```python
from build123d import *

# Parameters (mm, degrees)
SKETCH1_R           = 1.875
BOSS_EXTRUDE1_DEPTH = 15
SKETCH2_W           = 35
SKETCH2_H           = 2.286
CUT_EXTRUDE1_DEPTH  = 1.778
SKETCH7_W           = 23.625
SKETCH7_H           = 2.286
CUT_EXTRUDE6_DEPTH  = 5
SKETCH3_R           = 3.302
CUT_EXTRUDE2_DEPTH  = 3.556
SKETCH4_R           = 3.302
CUT_EXTRUDE3_DEPTH  = 3.302
SKETCH5_W           = 35
SKETCH5_H           = 15
CUT_EXTRUDE4_DEPTH  = 0.762
CUT_EXTRUDE5_DEPTH  = 73.293856534
FILLET1_R           = 3
FILLET2_R           = 1


with BuildPart() as part:
    # Sketch1 → Boss-Extrude1 (new body)
    with BuildSketch(Plane(origin=(0, 0, 0), x_dir=(1, 0, 0), z_dir=(0, 1, 0))):
        with BuildLine():
            Line((-60.8, 0), (0, 0))
            Line((0, 0), (0, 35))
            Line((0, 35), (-16.036868781, 35))
            Line((-16.036868781, 35), (-16.036868781, 15))
            Line((-16.036868781, 15), (-60.8, 15))
            ThreePointArc((-60.8, 15), (-61.45243439, 7.5), (-60.8, 0))
        make_face()
        with Locations(Location((-8.01843439, 7.5, 0), (0, 0, 270))):
            Circle(SKETCH1_R, mode=Mode.SUBTRACT)
    extrude(amount=BOSS_EXTRUDE1_DEPTH)

    # Sketch2 → Cut-Extrude1 (cut)
    with BuildSketch(Plane(origin=(0, 0, 0), x_dir=(0, 0, -1), z_dir=(1, 0, 0))):
        with BuildLine():
            Line((22.486, 12.716), (22.486, 15))
            Line((22.486, 15), (0, 15))
            Line((0, 15), (0, 4.043897552))
            Line((0, 4.043897552), (18.893897552, 4.043897552))
            ThreePointArc((18.893897552, 4.043897552), (27.179308025, 5.691968164), (22.486, 12.716))
        make_face()
        with Locations((17.5, 1.143)):
            Rectangle(SKETCH2_W, SKETCH2_H)
    extrude(amount=-CUT_EXTRUDE1_DEPTH, mode=Mode.SUBTRACT)

    # Sketch7 → Cut-Extrude6 (cut)
    with BuildSketch(Plane(origin=(-1.778, 0, 0), x_dir=(0, 0, -1), z_dir=(1, 0, 0))):
        with Locations((23.1875, 1.143)):
            Rectangle(SKETCH7_W, SKETCH7_H)
    extrude(amount=-CUT_EXTRUDE6_DEPTH, mode=Mode.SUBTRACT)

    # Sketch3 → Cut-Extrude2 (cut)
    with BuildSketch(Plane(origin=(-1.778, 0, 0), x_dir=(0, 0, -1), z_dir=(1, 0, 0))):
        with Locations((22.486, 7.636)):
            Circle(SKETCH3_R)
    extrude(amount=-CUT_EXTRUDE2_DEPTH, mode=Mode.SUBTRACT)

    # Sketch4 → Cut-Extrude3 (cut)
    with BuildSketch(Plane(origin=(0, 0, -15), x_dir=(-1, 0, 0), z_dir=(0, 0, -1))):
        with Locations((43.57843439, 7.5)):
            Circle(SKETCH4_R)
    extrude(amount=-CUT_EXTRUDE3_DEPTH, mode=Mode.SUBTRACT)

    # Sketch5 → Cut-Extrude4 (cut)
    with BuildSketch(Plane(origin=(0, 0, 0), x_dir=(0, 0, -1), z_dir=(1, 0, 0))):
        with Locations((17.5, 7.5)):
            Rectangle(SKETCH5_W, SKETCH5_H)
    extrude(amount=-CUT_EXTRUDE4_DEPTH, mode=Mode.SUBTRACT)

    # Sketch6 → Cut-Extrude5 (cut, through all)
    with BuildSketch(Plane(origin=(0, 15, 0), x_dir=(1, 0, 0), z_dir=(0, 1, 0))):
        with BuildLine():
            Line((-8.262, 0), (-0.762, 0))
            Line((-0.762, 0), (-0.762, 7.5))
            ThreePointArc((-0.762, 7.5), (-2.958699141, 2.196699141), (-8.262, 0))
        make_face()
    extrude(amount=-CUT_EXTRUDE5_DEPTH, mode=Mode.SUBTRACT)

    # Fillet1
    fillet1_edges = [part.edges().sort_by_distance(p)[0] for p in [
        (-60.8, 7.5, 0),
        (-60.8, 7.5, -15),
        (-16.036868781, 7.5, -15),
        (-16.036868781, 7.5, -35),
        (-0.762, 8.643, -35),
    ]]
    fillet(fillet1_edges, radius=FILLET1_R)

    # Fillet2
    fillet2_edges = [part.edges().sort_by_distance(p)[0] for p in [
        (-1.778, 0, -7.552841941),
        (-4.521670528, 15, -0.99923578),
        (-4.521670528, 0, -0.99923578),
        (-61.45243439, 0, -7.5),
        (-61.45243439, 15, -7.5),
        (-33.231623045, 0, 0),
        (-38.619057435, 0, -15),
        (-16.036868781, 0, -25),
        (-15.158189125, 0, -34.121320344),
        (-60.201042042, 0, -0.763749534),
        (-60.201042042, 0, -14.236250466),
        (-38.619057435, 15, -15),
        (-0.762, 15, -27.243),
        (-8.39943439, 15, -35),
        (-16.036868781, 15, -25),
        (-33.231623045, 15, 0),
        (-15.158189125, 15, -34.121320344),
        (-1.640679656, 15, -34.121320344),
        (-60.201042042, 15, -0.763749534),
        (-60.201042042, 15, -14.236250466),
        (-16.915548437, 0, -15.878679656),
        (-16.915548437, 15, -15.878679656),
        (-8.01843439, 0, -9.375),
        (-8.01843439, 15, -9.375),
        (-1.778, 15, -13.108341941),
        (-1.27, 15, -22.486),
        (-9.90743439, 0, -35),
        (-4.278, 0, -11.375),
        (-6.778, 0, -23.1875),
        (-1.778, 1.143, -11.375),
    ]]
    fillet(fillet2_edges, radius=FILLET2_R)


solid = part.part
```
For this review, take the finished solid that the model builds, in its own axes (mm). A direction names the side the tool comes from. Round coordinates to 2 decimals unless told otherwise and drop trailing zeros. Write each loop counter-clockwise with the first axis right and the second up, starting at its lowest first coordinate (ties: lowest second). Pieces come first, ordered by that corner, then holes. Notation, with made-up numbers: (45, 77.5) -> (70, 77.5) arc R10 cw to (70, 93.5) -> close; hole circle Ø6 at (-25, -36.75). An arc over 180 degrees is marked (long way). Use one line per item in the form item = value.
1) Take a section at B-B, the plane z = -25. Write out the cut boundary in (x, y), and give its area (3 significant figures).
Found:
outline = (-16.04, 1) arc R1 ccw to (-15.04, 0) -> (-7.78, 0) arc R1 ccw to (-6.78, 1) -> (-6.78, 2.29) -> (-0.76, 2.29) -> (-0.76, 3.22) -> (-1.78, 3.22) -> (-1.78, 5.5) -> (-5.33, 5.5) -> (-5.33, 9.78) -> (-1.78, 9.78) -> (-1.78, 12.05) -> (-0.76, 12.05) -> (-0.76, 14) arc R1 ccw to (-1.76, 15) -> (-15.04, 15) arc R1 ccw to (-16.04, 14) -> close
area = 190 mm2
2) Tool access review of faces 5 (the flat face through (-6.778, 2, -23)), 6 (the flat face through (-44, 8, -11.698)), 7 (the flat face through (-1.778, 2, -7)), 8 (the flat face through (-38, 7, -15)): name each direction out of +Z, -Z, +X, -X, +Y, -Y from which nothing blocks a thin tool from reaching the whole face with its end or side.
Found:
face_5 = -Z, +X, -Y
face_6 = -Z
face_7 = +Z, -Z, +X, -Y
face_8 = -Z, -X, +Y, -Y
3) Clearance check with flat-ended pins moving along their axes: pin 1 (6.5 mm diameter, centred on x = -4, z = -20, fed in from -Y); pin 2 (1.1 mm diameter, centred on x = -1, y = 13.5, fed in from +Z); pin 3 (1.5 mm diameter, centred on y = 10.5, z = -20, fed in from +X). State where each tip first meets the part, or that it passes through.
Found:
pin_1 = 0.15
pin_2 = -22.49
pin_3 = -1.78
4) Take a section at A-A, the plane x = -31. Write out the cut boundary in (y, z), and give its area (3 significant figures).
Found:
outline = (0, -14) arc R1 ccw to (1, -15) -> (14, -15) arc R1 ccw to (15, -14) -> (15, -1) arc R1 ccw to (14, 0) -> (1, 0) arc R1 ccw to (0, -1) -> close
area = 224 mm2
5) To check wall thickness, follow L1, parallel to Z at x = -8, y = 6; L2, parallel to X at y = 3.5, z = -31.5; L3, parallel to X at y = 1, z = -24. State the ranges of each line that lie inside material, in increasing order. Write a range as from..to.
Found:
L1 = -35..-9.37, -5.63..0
L2 = -16.04..-0.76
L3 = -16.04..-6.78
6) Mouldability with a two-part tool opening along Z and no side actions: class faces 1 (the cylindrical face through (-7.936, 7.409, -9.373)), 2 (the flat face through (-5.334, 8, -22)), 3 (the cylindrical face through (-1.66, 8.22, -34.14)), 4 (the cylindrical face through (-42.863, 4.277, -13.372)) as +Z half, -Z half, draft (parallel to the pull), parting line (faces both ways), or undercut.
Found:
face_1 = undercut
face_2 = undercut
face_3 = -Z half
face_4 = draft
